Answer from the drawing. Dimensions are ordinates in mm from the lowest x, y and z of the part. Coordinates: 2 decimals unless noted, no trailing zeros. Loops run counter-clockwise (first coordinate to the right, second up) from the corner with the lowest first, then second, coordinate; pieces in that order, holes last.
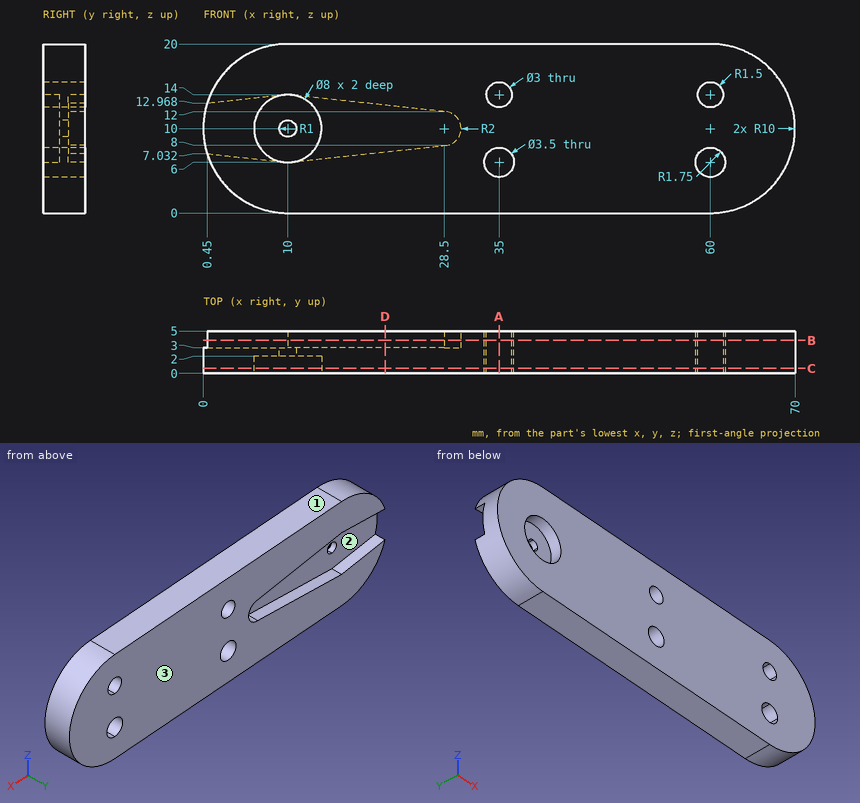
Item 1: Determine the mould class of the marked faces 1, 2 and 3 for opening direction Z: released by +Z, released by -Z, zero draft, split by the parting line, or undercut.
Numbers:
face 1: released by +Z
face 2: undercut
face 3: zero draft
Item 2: A cutting plane is placed at D-D on x = 21.5. Determine the outline of the cut face in (y, z).
Numbers:
outline: (0, 0) - (5, 0) - (5, 7.24) - (3, 7.24) - (3, 12.76) - (5, 12.76) - (5, 20) - (0, 20) - close
Item 3: A cutting plane is placed at A-A on x = 35. Determine the outline of the cut face in (y, z).
Numbers:
outline: (0, 0) - (5, 0) - (5, 4.25) - (0, 4.25) - close; (0, 7.75) - (5, 7.75) - (5, 12.5) - (0, 12.5) - close; (0, 15.5) - (5, 15.5) - (5, 20) - (0, 20) - close
Item 4: Given pin 1 (6.5 mm diameter, centred on x = 13.5, z = 8.5, fed in from +Y), flat-ended and moving along its own axis, determine where the tip first touches the part or whether it passes through.
Numbers:
pin 1: stops at y = 5
Item 5: A cutting plane is placed at C-C on y = 0.6. Determine the outline of the cut face in (x, z), then the cut area to 3 significant figures.
Numbers:
outline: (10, 0) - (60, 0) arc R10 ccw to (60, 20) - (10, 20) arc R10 ccw to start; hole circle Ø8 at (10, 10); hole circle Ø3.5 at (35, 6); hole circle Ø3 at (35, 14); hole circle Ø3.5 at (60, 6); hole circle Ø3 at (60, 14)
area: 1,230 mm2
Item 6: Find the intervals of material crossed by line 1 along X through (y, z) = (0.45, 7.25) (1 decimal); line 2 along X through (y, z) = (1.7, 9.25); line 3 along Z through (x, y) = (27, 3.35), in increasing order.
Numbers:
line 1: x = 0.4 to 7.1, 12.9 to 33.8, 36.2 to 58.8, 61.2 to 69.6
line 2: x = 0.03 to 6.07, 13.93 to 69.97
line 3: z = 0 to 7.84, 12.16 to 20
Item 7: A cutting plane is placed at B-B on y = 3.9. Determine the outline of the cut face in (x, z), then the cut area to 4 significant figures.
Numbers:
outline: (0.45, 7.03) arc R10 ccw to (10, 0) - (60, 0) arc R10 ccw to (60, 20) - (10, 20) arc R10 ccw to (0.45, 12.97) - (10, 14) - (28.5, 12) arc R2 cw to (28.5, 8) - (10, 6) - close; hole circle Ø3.5 at (35, 6); hole circle Ø3 at (35, 14); hole circle Ø3.5 at (60, 6); hole circle Ø3 at (60, 14)
area: 1,095 mm2
